Work out the finished part from the listing and answer in its coordinate system (mm). A direction names the side the tool comes from. Round coordinates to 2 decimals unless told otherwise and drop trailing zeros. Write each loop counter-clockwise with the first axis right and the second up, starting at its lowest first coordinate (ties: lowest second). Pieces come first, ordered by that corner, then holes. Notation, with made-up numbers: (-39, 3) -> (-28, 3) arc R36 cw to (-28, 40) -> close; hole circle Ø9 at (50.5, 18.25). An arc over 180 degrees is marked (long way). One line per item, written item: value.
```python
from build123d import *

# Parameters (mm, degrees)
BOSS_EXTRUDE1_DEPTH = 41.8
CHAMFER1_SIZE       = 0.4
BOSS_EXTRUDE2_DEPTH = 1
CHAMFER2_SIZE       = 0.4


with BuildPart() as part:
    # Sketch1 → Boss-Extrude1 (new body)
    with BuildSketch(Plane(origin=(0, 0, 0), x_dir=(1, 0, 0), z_dir=(0, 1, 0))):
        with BuildLine():
            Line((-2.482438317, -3.2), (2.482438317, -3.2))
            ThreePointArc((2.482438317, -3.2), (4.05, 0), (2.482438317, 3.2))
            Line((2.482438317, 3.2), (-2.482438317, 3.2))
            ThreePointArc((-2.482438317, 3.2), (-4.05, 0), (-2.482438317, -3.2))
        make_face()
    extrude(amount=BOSS_EXTRUDE1_DEPTH)

    # Chamfer1
    chamfer1_edges = [part.edges().sort_by_distance(p)[0] for p in [
        (0, 41.8, -3.2),
        (-4.05, 41.8, 0),
        (4.05, 41.8, 0),
        (0, 41.8, 3.2),
        (4.05, 0, 0),
        (0, 0, 3.2),
        (-4.05, 0, 0),
        (0, 0, -3.2),
    ]]
    chamfer(chamfer1_edges, length=CHAMFER1_SIZE)

    # Sketch2 → Boss-Extrude2 (add)
    with BuildSketch(Plane(origin=(0, 22.2, 0), x_dir=(1, 0, 0), z_dir=(0, 1, 0))):
        with BuildLine():
            Line((-5.075431016, -3.2), (5.075431016, -3.2))
            ThreePointArc((5.075431016, -3.2), (6, 0), (5.075431016, 3.2))
            Line((5.075431016, 3.2), (-5.075431016, 3.2))
            ThreePointArc((-5.075431016, 3.2), (-6, 0), (-5.075431016, -3.2))
        make_face()
    extrude(amount=-BOSS_EXTRUDE2_DEPTH)

    # Chamfer2
    chamfer2_edges = [part.edges().sort_by_distance(p)[0] for p in [
        (-6, 22.2, 0),
        (-6, 21.2, 0),
        (6, 21.2, 0),
        (6, 22.2, 0),
    ]]
    chamfer(chamfer2_edges, length=CHAMFER2_SIZE)


solid = part.part
```
(1) Find section A-A on y = 28.5. Give the vertices of the cut face in (x, z), plus the area to 3 significant figures.
Reported:
outline: (-2.48, -3.2) -> (2.48, -3.2) arc R4.05 ccw to (2.48, 3.2) -> (-2.48, 3.2) arc R4.05 ccw to start
area: 45.8 mm2
(2) A tool of negligible diameter and unlimited length cuts with its end or side. For faces 1 (the face through (-4.05, 10.65, -0.05)), 2 (the face through (4.4, 22.2, 0)), 3 (the face through (-4.05, 31.67, -0.05)), from which of +Z, -Z, +X, -X, +Y, -Y can it reach the whole face along a straight path? Write none if from no direction.
Reported:
face 1: -X, -Y
face 2: +X, +Y
face 3: -X, +Y
(3) Consider probe 1 along Y at (x, z) = (-4.5, -0.5); probe 2 along X at (y, z) = (3, 2.5); probe 3 along X at (y, z) = (14, 0.25). Determine where each line is inside the solid, lowest interval first.
Reported:
probe 1: y = 21.2 to 22.2
probe 2: x = -3.19 to 3.19
probe 3: x = -4.04 to 4.04
(4) Flat-ended cylindrical pins translate along their axes: pin 1 Ø3 at (y, z) = (36, -1.5) entering from +X; pin 2 Ø1 at (y, z) = (10, 1) entering from -X; pin 3 Ø1.6 at (x, z) = (-4.5, 0) entering from +Y. Find the tip coordinate at first contact, or state that the pin passes through.
Reported:
pin 1: stops at x = 4.05
pin 2: stops at x = -4.02
pin 3: stops at y = 41.75
